Design review of the part built by this model. Coordinates are the model's own, in mm. A direction names the side the tool comes from. Give positions to 0.01 mm unless a question says otherwise; leave off trailing zeros. Write each loop counter-clockwise with the first axis right and the second up, starting at its lowest first coordinate (ties: lowest second). Pieces come first, ordered by that corner, then holes. Notation, with made-up numbers: (-31.5, 69.5) -> (9.5, 69.5) arc R21 cw to (9.5, 105.5) -> close; hole circle Ø8 at (-35.75, 48). An arc over 180 degrees is marked (long way). Write each question's results on one line, items separated by ' | '. Start each with the question number.
(1) Take a section at C-C (y = 0.6). Count the separate pieces of the cut face and the enclosed holes in it, plus the area to 3 significant figures.
(2) Take a section at B-B (z = -77). State the section outline as (x, y) points.
(3) Mouldability with a two-part tool opening along Z and no side actions: class faces 1 (the face through (-73, 0, -200)), 2 (the face through (66.041, 0.789, -217.134)), 3 (the face through (-219.163, 0.789, -89.985)), 4 (the face through (-38.7, 0.8, -56.5)) as released by +Z, released by -Z, zero draft, split by the parting line, or undercut.
(4) To check wall thickness, follow probe 1 along X at (y, z) = (1.1, -138); probe 2 along Z at (x, y) = (-152, 1); probe 3 along X at (y, z) = (0.45, -177). State the ranges of each line that lie inside material, in increasing order.
(5) Clearance check with flat-ended pins moving along their axes: pin 1 (2 mm diameter, centred on x = -132.44, z = -21.35, fed in from -Y); pin 2 (0.5 mm diameter, centred on x = -30, y = 0.5, fed in from -Z); pin 3 (0.8 mm diameter, centred on y = 1, z = -248, fed in from -X); pin 4 (0.5 mm diameter, centred on y = 0.5, z = -95.5, fed in from +X). State where each tip first meets the part, or that it passes through.
(6) Take a section at A-A (x = -67). State the section outline as (y, z) points.
(7) For faces 5 (the face through (-102.4, 0.79, -56.32)), 6 (the face through (-213.475, 0.789, -206.266)), 7 (the face through (-143.478, 0.789, -34.396)), 8 (the face through (13.594, 0.789, -3.108)), 9 (the face through (2.95, 0.79, -34.3)), list the 3-axis set-ups (+Z, -Z, +X, -X, +Y, -Y) from which the entire face can be reached by the end or side of a thin tool; tool diameter is ignored.
from build123d import *

# Parameters (mm, degrees)
SKETCH1_R           = 1.75
BOSS_EXTRUDE1_DEPTH = 1.6
SKETCH3_R           = 8
CUT_EXTRUDE1_DEPTH  = 1.6


with BuildPart() as part:
    # Sketch1 → Boss-Extrude1 (new body)
    with BuildSketch(Plane(origin=(0, 0, 0), x_dir=(1, 0, 0), z_dir=(0, 1, 0))):
        with BuildLine():
            Line((24.696313384, 21.403189927), (-19.414899465, 47.563680085))
            ThreePointArc((-19.414899465, 47.563680085), (-20.786874634, 49.384536896), (-20.482680557, 51.644028288))
            Line((-20.482680557, 51.644028288), (17.162414168, 116.847245007))
            ThreePointArc((17.162414168, 116.847245007), (19.546471274, 118.676596366), (22.525800971, 118.28436017))
            Line((22.525800971, 118.28436017), (70.987796177, 90.304814192))
            ThreePointArc((70.987796177, 90.304814192), (77.999004119, 90.304814192), (81.50460809, 96.376698381))
            Line((81.50460809, 96.376698381), (81.50460809, 182.02519482))
            ThreePointArc((81.50460809, 182.02519482), (80.873629228, 187.452491566), (79.01435205, 192.590270527))
            Line((79.01435205, 192.590270527), (69.144094326, 212.364639151))
            ThreePointArc((69.144094326, 212.364639151), (65.989183491, 217.196365343), (61.81193417, 221.177524531))
            Line((61.81193417, 221.177524531), (44.99314954, 233.854205885))
            Line((44.99314954, 233.854205885), (-23.199197227, 273.225075648))
            ThreePointArc((-23.199197227, 273.225075648), (-28.860512938, 273.225075648), (-31.691170793, 268.322232423))
            Line((-31.691170793, 268.322232423), (-31.691170793, 207.371759387))
            ThreePointArc((-31.691170793, 207.371759387), (-32.56985045, 205.250439044), (-34.691170793, 204.371759387))
            Line((-34.691170793, 204.371759387), (-106.595635326, 204.371759387))
            ThreePointArc((-106.595635326, 204.371759387), (-108.71695567, 205.250439044), (-109.595635326, 207.371759387))
            Line((-109.595635326, 207.371759387), (-109.595635326, 268.322232423))
            ThreePointArc((-109.595635326, 268.322232423), (-112.426293182, 273.225075648), (-118.087608892, 273.225075648))
            Line((-118.087608892, 273.225075648), (-186.279955659, 233.854205885))
            Line((-186.279955659, 233.854205885), (-204.21495553, 220.336208987))
            ThreePointArc((-204.21495553, 220.336208987), (-207.400637767, 217.300070339), (-209.806657286, 213.615266508))
            Line((-209.806657286, 213.615266508), (-217.247579174, 198.707901735))
            ThreePointArc((-217.247579174, 198.707901735), (-221.386722215, 187.270122423), (-222.791414209, 175.187815477))
            Line((-222.791414209, 175.187815477), (-222.791414209, 96.376698381))
            ThreePointArc((-222.791414209, 96.376698381), (-219.069332913, 89.929864467), (-211.625170321, 89.929864467))
            Line((-211.625170321, 89.929864467), (-163.512384372, 117.707794386))
            ThreePointArc((-163.512384372, 117.707794386), (-160.504762554, 118.10375531), (-158.098066116, 116.257032182))
            Line((-158.098066116, 116.257032182), (-120.496410943, 51.129054973))
            ThreePointArc((-120.496410943, 51.129054973), (-120.196709676, 48.852597838), (-121.594487155, 47.030978762))
            Line((-121.594487155, 47.030978762), (-165.983119503, 21.403189927))
            Line((-165.983119503, 21.403189927), (-174.676412504, 16.182853027))
            ThreePointArc((-174.676412504, 16.182853027), (-176.124776412, 13.818668342), (-175.016914475, 11.277060748))
            Line((-175.016914475, 11.277060748), (-168.860075369, 6.304549502))
            Line((-168.860075369, 6.304549502), (-141.286806119, 0))
            Line((-141.286806119, 0), (0, 0))
            Line((0, 0), (27.57326925, 6.304549502))
            Line((27.57326925, 6.304549502), (33.730108356, 11.277060748))
            ThreePointArc((33.730108356, 11.277060748), (34.837970293, 13.818668342), (33.389606385, 16.182853027))
            Line((33.389606385, 16.182853027), (24.696313384, 21.403189927))
        make_face()
        with Locations(Location((-123.091146174, 191.349343748, 0), (0, 0, 270))):
            Circle(SKETCH1_R, mode=Mode.SUBTRACT)
        with Locations(Location((-216.641081117, 98.036380822, 0), (0, 0, 270))):
            Circle(SKETCH1_R, mode=Mode.SUBTRACT)
        with Locations(Location((-18.645659945, 191.349343748, 0), (0, 0, 90))):
            Circle(SKETCH1_R, mode=Mode.SUBTRACT)
        with Locations(Location((74.914274997, 98.036380822, 0), (0, 0, 90))):
            Circle(SKETCH1_R, mode=Mode.SUBTRACT)
        with Locations(Location((-9.245725003, 21.35, 0), (0, 0, 270))):
            Circle(SKETCH1_R, mode=Mode.SUBTRACT)
        with Locations(Location((-132.441081117, 21.35, 0), (0, 0, 270))):
            Circle(SKETCH1_R, mode=Mode.SUBTRACT)
        with Locations(Location((-150.641414209, 135.049343748, 0), (0, 0, 270))):
            Circle(SKETCH1_R, mode=Mode.SUBTRACT)
        with Locations(Location((8.91460809, 135.049343748, 0), (0, 0, 270))):
            Circle(SKETCH1_R, mode=Mode.SUBTRACT)
        with Locations(Location((68.354340055, 202.349343748, 0), (0, 0, 270))):
            Circle(SKETCH1_R, mode=Mode.SUBTRACT)
        with Locations(Location((-11.691170793, 259.371759387, 0), (0, 0, 270))):
            Circle(SKETCH1_R, mode=Mode.SUBTRACT)
        with Locations(Location((-129.595635326, 259.371759387, 0), (0, 0, 270))):
            Circle(SKETCH1_R, mode=Mode.SUBTRACT)
        with Locations(Location((-209.641146174, 202.349343748, 0), (0, 0, 270))):
            Circle(SKETCH1_R, mode=Mode.SUBTRACT)
        Polygon((-31.555725003, 63.222149708), (-46.022445575, 49.606380822), (-95.264360544, 49.606380822), (-109.731081117, 63.222149708), (-109.731081117, 137.774232151), (-112.861146174, 137.774232151), (-112.861146174, 182.049343748), (-28.425659945, 182.049343748), (-28.425659945, 137.774232151), (-31.555725003, 137.774232151), align=None, mode=Mode.SUBTRACT)
    extrude(amount=BOSS_EXTRUDE1_DEPTH)

    # Sketch3 → Cut-Extrude1 (cut)
    with BuildSketch(Plane(origin=(0, 1.6, 0), x_dir=(1, 0, 0), z_dir=(0, 1, 0))):
        with Locations(Location((43.415663258, 132.362201431, 0), (0, 0, 270))):
            Circle(SKETCH3_R)
    extrude(amount=-CUT_EXTRUDE1_DEPTH, mode=Mode.SUBTRACT)


solid = part.part
Report:
1) separate pieces: 1 | enclosed holes: 14 | area: 43,800 mm2
2) outline: (-135.43, 0) -> (-109.73, 0) -> (-109.73, 1.6) -> (-135.43, 1.6) -> close; (-31.56, 0) -> (-5.84, 0) -> (-5.84, 1.6) -> (-31.56, 1.6) -> close
3) face 1: zero draft | face 2: released by -Z | face 3: released by +Z | face 4: undercut
4) probe 1: -222.79 to -112.86, -28.43 to 37.74, 49.09 to 81.5 | probe 2: -253.65 to -136.15, -133.95 to -105.69, -29.48 to -2.45 | probe 3: -222.76 to -112.86, -28.43 to 81.5
5) pin 1: through | pin 2: z = -272.59 | pin 3: x = -162.47 | pin 4: x = 81.48
6) outline: (0, -204.37) -> (1.6, -204.37) -> (1.6, -182.05) -> (0, -182.05) -> close; (0, -49.61) -> (1.6, -49.61) -> (1.6, 0) -> (0, 0) -> close
7) face 5: +Y, -Y | face 6: -Z, -X, +Y, -Y | face 7: -X, +Y, -Y | face 8: +Z, +X, +Y, -Y | face 9: +X, +Y, -Y
